from build123d import *

# Parameters (mm, degrees)
CYLINDER008_R               = 2
CYLINDER008_DEPTH           = 10
BOX_W                       = 10
BOX_H                       = 4
BOX_DEPTH                   = 2
BOX_PLACEMENT_ANGLE         = 60
ARRAY001_COUNT              = 3
CYLINDER007_W               = 15
CYLINDER007_H               = 2
CYLINDER007_ANGLE           = 60
CYLINDER007_PLACEMENT_ANGLE = 95
CYLINDER006_W               = 19
CYLINDER006_H               = 2
CYLINDER006_ANGLE           = 60
CYLINDER006_PLACEMENT_ANGLE = 95
CYLINDER005_W               = 15
CYLINDER005_H               = 2
CYLINDER005_ANGLE           = 60
CYLINDER005_PLACEMENT_ANGLE = 211
CYLINDER004_W               = 19
CYLINDER004_H               = 2
CYLINDER004_ANGLE           = 60
CYLINDER004_PLACEMENT_ANGLE = 211
CYLINDER003_W               = 15
CYLINDER003_H               = 2
CYLINDER003_ANGLE           = 60
CYLINDER003_PLACEMENT_ANGLE = -35
CYLINDER002_W               = 19
CYLINDER002_H               = 2
CYLINDER002_ANGLE           = 60
CYLINDER002_PLACEMENT_ANGLE = -35
SKETCH001_R                 = 5.198312
PAD_DEPTH                   = 4
ARRAY_COUNT                 = 3


with BuildPart() as cilindro007:
    # Cylinder008 → Cylinder008 (new body)
    with BuildSketch(Plane(origin=(-0.25, 15, -4), x_dir=(1, 0, 0), z_dir=(0, 0, 1))):
        Circle(CYLINDER008_R)
    extrude(amount=CYLINDER008_DEPTH)


with BuildPart() as array001:
    # Box → Box (new body)
    with BuildSketch(Plane.XY):
        with Locations((5, 2)):
            Rectangle(BOX_W, BOX_H)
    extrude(amount=BOX_DEPTH)


with BuildPart() as array001_1:
    # Box placement: moved
    add(array001.part.moved(Location((-3, 6, 0))).rotate(Axis((-3, 6, 0), (0, 0, 1)), BOX_PLACEMENT_ANGLE))

    # Array001: Array001 ×3 about axis
    array001_axis = Axis((-12.5, -6.5, 0), (0, 0, 1))


with BuildPart() as array001_2:
    add(array001_1.part)
    for i in range(1, ARRAY001_COUNT):
        add(array001_1.part.rotate(array001_axis, i * 360 / ARRAY001_COUNT))


with BuildPart() as cilindro006:
    # Cylinder007 → Cylinder007 (revolve)
    with BuildSketch(Plane.XZ):
        with Locations((7.5, 1)):
            Rectangle(CYLINDER007_W, CYLINDER007_H)
    revolve(axis=Axis((0, 0, 0), (0, 0, 1)), revolution_arc=CYLINDER007_ANGLE)


with BuildPart() as cilindro006_1:
    # Cylinder007 placement: moved
    add(cilindro006.part.moved(Location((-12.5, -6.5, 0))).rotate(Axis((-12.5, -6.5, 0), (0, 0, 1)), CYLINDER007_PLACEMENT_ANGLE))


with BuildPart() as cut003:
    # Cylinder006 → Cylinder006 (revolve)
    with BuildSketch(Plane.XZ):
        with Locations((9.5, 1)):
            Rectangle(CYLINDER006_W, CYLINDER006_H)
    revolve(axis=Axis((0, 0, 0), (0, 0, 1)), revolution_arc=CYLINDER006_ANGLE)


with BuildPart() as cut003_1:
    # Cylinder006 placement: moved
    add(cut003.part.moved(Location((-12.5, -6.5, 0))).rotate(Axis((-12.5, -6.5, 0), (0, 0, 1)), CYLINDER006_PLACEMENT_ANGLE))

    # Cut003: cut Cilindro006
    add(cilindro006_1.part, mode=Mode.SUBTRACT)


with BuildPart() as cilindro004:
    # Cylinder005 → Cylinder005 (revolve)
    with BuildSketch(Plane.XZ):
        with Locations((7.5, 1)):
            Rectangle(CYLINDER005_W, CYLINDER005_H)
    revolve(axis=Axis((0, 0, 0), (0, 0, 1)), revolution_arc=CYLINDER005_ANGLE)


with BuildPart() as cilindro004_1:
    # Cylinder005 placement: moved
    add(cilindro004.part.moved(Location((-12.5, -6.5, 0))).rotate(Axis((-12.5, -6.5, 0), (0, 0, 1)), CYLINDER005_PLACEMENT_ANGLE))


with BuildPart() as cut002:
    # Cylinder004 → Cylinder004 (revolve)
    with BuildSketch(Plane.XZ):
        with Locations((9.5, 1)):
            Rectangle(CYLINDER004_W, CYLINDER004_H)
    revolve(axis=Axis((0, 0, 0), (0, 0, 1)), revolution_arc=CYLINDER004_ANGLE)


with BuildPart() as cut002_1:
    # Cylinder004 placement: moved
    add(cut002.part.moved(Location((-12.5, -6.5, 0))).rotate(Axis((-12.5, -6.5, 0), (0, 0, 1)), CYLINDER004_PLACEMENT_ANGLE))

    # Cut002: cut Cilindro004
    add(cilindro004_1.part, mode=Mode.SUBTRACT)


with BuildPart() as cilindro002:
    # Cylinder003 → Cylinder003 (revolve)
    with BuildSketch(Plane.XZ):
        with Locations((7.5, 1)):
            Rectangle(CYLINDER003_W, CYLINDER003_H)
    revolve(axis=Axis((0, 0, 0), (0, 0, 1)), revolution_arc=CYLINDER003_ANGLE)


with BuildPart() as cilindro002_1:
    # Cylinder003 placement: moved
    add(cilindro002.part.moved(Location((-12.5, -6.5, 0))).rotate(Axis((-12.5, -6.5, 0), (0, 0, 1)), CYLINDER003_PLACEMENT_ANGLE))


with BuildPart() as fusion:
    # Cylinder002 → Cylinder002 (revolve)
    with BuildSketch(Plane.XZ):
        with Locations((9.5, 1)):
            Rectangle(CYLINDER002_W, CYLINDER002_H)
    revolve(axis=Axis((0, 0, 0), (0, 0, 1)), revolution_arc=CYLINDER002_ANGLE)


with BuildPart() as fusion_1:
    # Cylinder002 placement: moved
    add(fusion.part.moved(Location((-12.5, -6.5, 0))).rotate(Axis((-12.5, -6.5, 0), (0, 0, 1)), CYLINDER002_PLACEMENT_ANGLE))

    # Cut001: cut Cilindro002
    add(cilindro002_1.part, mode=Mode.SUBTRACT)

    # Fusion: union Cut003, Cut002
    add(cut003_1.part)
    add(cut002_1.part)


with BuildPart() as cut004:
    # Sketch001 → Pad (new body)
    with BuildSketch(Plane.XY):
        with Locations((-0.149011, 15.05543)):
            Circle(SKETCH001_R)
        with BuildLine():
            ThreePointArc((0.265943, -4.477766), (-6.03588, 4.72153), (-17.151991, 5.600213))
            Line((-21.656212, 13.370653), (-17.151991, 5.600213))
            ThreePointArc((-7.750284, 14.849869), (-14.824787, 15.252835), (-21.656212, 13.370653))
            ThreePointArc((-7.750284, 14.849869), (-3.935994, 8.461466), (3.504091, 8.386363))
            ThreePointArc((9.244463, -4.477766), (7.439427, 2.429601), (3.504091, 8.386363))
            Line((0.265943, -4.477766), (9.244463, -4.477766))
        make_face()
    extrude(amount=PAD_DEPTH)

    # Array: Cut004 ×3 about axis
    array_axis = Axis((-12.5, -6.5, 0), (0, 0, 1))


with BuildPart() as cut004_1:
    add(cut004.part)
    for i in range(1, ARRAY_COUNT):
        add(cut004.part.rotate(array_axis, i * 360 / ARRAY_COUNT))

    # Fusion001: union Fusion
    add(fusion_1.part)

    # Fusion002: union Array001
    add(array001_2.part)

    # Cut004: cut Cilindro007
    add(cilindro007.part, mode=Mode.SUBTRACT)


with BuildPart() as cut004_2:
    # Cut004 placement: moved
    add(cut004_1.part.moved(Location((0, 1, 0))))


solid = cut004_2.part
Geometry: final body of the model. Coordinates: model frame, mm. A direction names the side the tool comes from. Coordinates: 2 decimals unless noted, no trailing zeros. Write each loop counter-clockwise with the first axis right and the second up, starting at its lowest first coordinate (ties: lowest second). Pieces come first, ordered by that corner, then holes. Notation, with made-up numbers: (46.5, -9) - (59.5, -9) arc R27 cw to (59.5, 19) - close; hole circle Ø4 at (-29.75, 26.5). An arc over 180 degrees is marked (long way). Return JSON: item names as keys, results as strings.
Item 1: Reachability of faces 4 (the face through (-31, -3.523, 1)), 5 (the face through (-14.84, -27.22, 1.97)), 6 (the face through (-22.85, 8.38, 2.42)) from +Z, -Z, +X, -X, +Y, -Y: full face, straight path, thin tool, end or side. Return the list, or none.
Completed:
{"face 4": "+Z, -Z", "face 5": "+Z, -Z, -Y", "face 6": "+Z"}
Item 2: Section query A-A (x = -11). Output: boundary loops of the cut face in (y, z).
Completed:
{"outline": "(-27.3, 0) - (-18.35, 0) - (-18.35, 4) - (-27.3, 4) - close; (7.37, 0) - (16.32, 0) - (16.32, 4) - (7.37, 4) - close"}
Item 3: Section query C-C (x = -37). Output: boundary loops of the cut face in (y, z), and give its area (3 significant figures).
Completed:
{"outline": "(-10.77, 0) - (-0.39, 0) - (-0.39, 4) - (-10.77, 4) - close", "area": "41.5 mm2"}
Item 4: Pull-direction query (Y, two-part tool) for faces 1 (the face through (-1.4, 9.77, 0.99)), 2 (the face through (-5, -17, 4)), 3 (the face through (-30.235, -18.309, 1.972)); classes: +Y half, -Y half, draft (parallel to the pull), parting line (faces both ways), or undercut.
Completed:
{"face 1": "undercut", "face 2": "draft", "face 3": "-Y half"}
Item 5: Section query B-B (z = 3.4). Output: boundary loops of the cut face in (x, y).
Completed:
{"outline": "circle Ø10.4 at (-37.34, -5.58); (-33.39, 0.92) arc R7.6 cw to (-33.36, -12.06) arc R21.85 ccw to (-25.13, -23.36) - (-20.65, -15.58) arc R12.93 cw to (-20.63, 4.54) - (-25.12, 12.32) arc R21.85 ccw to start; (-21.66, 14.37) - (-17.15, 6.6) arc R12.93 cw to (0.27, -3.48) - (9.24, -3.48) arc R21.85 ccw to (3.5, 9.39) arc R7.6 cw to (-7.75, 15.85) arc R21.85 ccw to start; (-21.62, -25.34) arc R21.85 ccw to (-7.61, -26.8) arc R7.6 cw to (3.61, -20.29) arc R21.85 ccw to (9.29, -7.51) - (0.31, -7.52) arc R12.93 cw to (-17.13, -17.57) - close; circle Ø10.4 at (-0.15, 16.06); circle Ø10.4 at (-0.01, -26.97); hole circle Ø4 at (-0.25, 16)"}
Item 6: Line query: L1, parallel to X at y = 5, z = 0.5; L2, parallel to Y at x = 3.5, z = 1.2; L3, parallel to Y at x = -10.5, z = 2.8. Output: solid intervals per line, ascending.
Completed:
{"L1": "x = -31.66 to -20.9, -4.92 to 6.66", "L2": "y = -30.81 to -23.14, -20.23 to 9.38, 12.35 to 19.76", "L3": "y = -27.26 to -18.28, 7.3 to 16.28"}
Item 7: Pin query (flat end, axial travel): pin 1 Ø1 at (x, z) = (-31, 1) entering from -Y; pin 2 Ø2 at (x, z) = (-8, 0.5) entering from +Y; pin 3 Ø0.6 at (x, z) = (-31.5, 0.5) entering from +Y; pin 4 Ø3 at (x, y) = (-0.25, 16) entering from +Z. Return the tip coordinate at first contact, or that it passes through.
Completed:
{"pin 1": "stops at y = -17.93", "pin 2": "stops at y = 16.09", "pin 3": "stops at y = 5.8", "pin 4": "passes through"}
Item 8: Section query D-D (y = -28.5). Output: boundary loops of the cut face in (x, z).
Completed:
{"outline": "(-4.98, 0) - (4.96, 0) - (4.96, 4) - (-4.98, 4) - close"}
